Build history of the part. All positions in model axes, mm. A direction names the side the tool comes from. Round coordinates to 2 decimals unless told otherwise and drop trailing zeros. Write each loop counter-clockwise with the first axis right and the second up, starting at its lowest first coordinate (ties: lowest second). Pieces come first, ordered by that corner, then holes.
from build123d import *

# Parameters (mm, degrees)
SKETCH1_W                = 40
SKETCH1_H                = 20
BOSS_EXTRUDE1_DEPTH      = 29
SKETCH2_W                = 54
SKETCH2_H                = 20
BOSS_EXTRUDE2_DEPTH      = 2.5
SKETCH3_W                = 40
SKETCH3_H                = 20
BOSS_EXTRUDE3_DEPTH      = 5.5
BOSS_EXTRUDE4_DEPTH      = 2
SKETCH5_R                = 6
BOSS_EXTRUDE5_DEPTH      = 2
SKETCH6_R                = 3
BOSS_EXTRUDE6_DEPTH      = 4
SKETCH7_R                = 2.05
CUT_EXTRUDE2_DEPTH       = 4
BOSS_EXTRUDE8_DEPTH      = 0.5
BOSS_EXTRUDE8_DEPTH_BACK = 0.5


with BuildPart() as part:
    # Sketch1 → Boss-Extrude1 (new body)
    with BuildSketch(Plane(origin=(0, 0, 0), x_dir=(1, 0, 0), z_dir=(0, 1, 0))):
        Rectangle(SKETCH1_W, SKETCH1_H)
    extrude(amount=BOSS_EXTRUDE1_DEPTH)

    # Sketch2 → Boss-Extrude2 (add)
    with BuildSketch(Plane(origin=(0, 29, 0), x_dir=(1, 0, 0), z_dir=(0, 1, 0))):
        Rectangle(SKETCH2_W, SKETCH2_H)
    extrude(amount=BOSS_EXTRUDE2_DEPTH)

    # Sketch3 → Boss-Extrude3 (add)
    with BuildSketch(Plane(origin=(0, 31.5, 0), x_dir=(1, 0, 0), z_dir=(0, 1, 0))):
        Rectangle(SKETCH3_W, SKETCH3_H)
    extrude(amount=BOSS_EXTRUDE3_DEPTH)

    # Sketch4 → Boss-Extrude4 (add)
    with BuildSketch(Plane(origin=(0, 37, 0), x_dir=(1, 0, 0), z_dir=(0, 1, 0))):
        with BuildLine():
            Line((-10.302888497, 5.203858548), (-10.302888497, 8.863863335))
            Line((-10.302888497, 8.863863335), (6.370537096, 8.863863335))
            ThreePointArc((6.370537096, 8.863863335), (14.138323544, 9.494784112), (20, 4.358898944))
            Line((20, 4.358898944), (20, -4.358898944))
            ThreePointArc((20, -4.358898944), (14.138323544, -9.494784112), (6.370537096, -8.863863335))
            Line((6.370537096, -8.863863335), (-10.302888497, -8.863863335))
            Line((-10.302888497, -8.863863335), (-10.302888497, -5.203858548))
            ThreePointArc((-10.302888497, -5.203858548), (-12.798836729, 0), (-10.302888497, 5.203858548))
        make_face()
    extrude(amount=BOSS_EXTRUDE4_DEPTH)

    # Sketch5 → Boss-Extrude5 (add)
    with BuildSketch(Plane(origin=(0, 39, 0), x_dir=(1, 0, 0), z_dir=(0, 1, 0))):
        with Locations((11, 0)):
            Circle(SKETCH5_R)
    extrude(amount=BOSS_EXTRUDE5_DEPTH)

    # Sketch6 → Boss-Extrude6 (add)
    with BuildSketch(Plane(origin=(0, 41, 0), x_dir=(1, 0, 0), z_dir=(0, 1, 0))):
        with Locations((11, 0)):
            Circle(SKETCH6_R)
    extrude(amount=BOSS_EXTRUDE6_DEPTH)

    # Sketch7 → Cut-Extrude2 (cut)
    with BuildSketch(Plane(origin=(0, 31.5, 0), x_dir=(1, 0, 0), z_dir=(0, 1, 0))):
        with Locations((-25, 5)):
            Circle(SKETCH7_R)
        with Locations((-25, -5)):
            Circle(SKETCH7_R)
        with Locations((25, 5)):
            Circle(SKETCH7_R)
        with Locations((25, -5)):
            Circle(SKETCH7_R)
    extrude(amount=-CUT_EXTRUDE2_DEPTH, mode=Mode.SUBTRACT)

    # Sketch8 → Boss-Extrude8 (add, two sides)
    with BuildSketch(Plane.XY) as boss_extrude8_sk:
        Polygon((-20, 34), (-27, 31.5), (-20, 31.5), align=None)
        Polygon((20, 31.5), (20, 34), (27, 31.5), align=None)
    extrude(amount=BOSS_EXTRUDE8_DEPTH)
    extrude(boss_extrude8_sk.sketch, amount=-BOSS_EXTRUDE8_DEPTH_BACK)


solid = part.part
1) Slice it at B-B (x = 25). Write the cut outline in (y, z).
Results:
outline: (29, -10) - (31.5, -10) - (31.5, -7.05) - (29, -7.05) - close; (29, -2.95) - (31.5, -2.95) - (31.5, -0.5) - (32.21, -0.5) - (32.21, 0.5) - (31.5, 0.5) - (31.5, 2.95) - (29, 2.95) - close; (29, 7.05) - (31.5, 7.05) - (31.5, 10) - (29, 10) - close
2) Slice it at C-C (y = 11.5). Write the cut outline in (x, z).
Results:
outline: (-20, -10) - (20, -10) - (20, 10) - (-20, 10) - close
3) Slice it at D-D (x = 12.5). Write the cut outline in (y, z), plus the area to 3 significant figures.
Results:
outline: (0, -10) - (37, -10) - (37, -9.89) - (39, -9.89) - (39, -5.81) - (41, -5.81) - (41, -2.6) - (45, -2.6) - (45, 2.6) - (41, 2.6) - (41, 5.81) - (39, 5.81) - (39, 9.89) - (37, 9.89) - (37, 10) - (0, 10) - close
area: 824 mm2
4) Pin check, flat tips, straight feed: pin 1 Ø6.5 at (x, z) = (25, 5) entering from -Y; pin 2 Ø6.5 at (x, z) = (25, -5) entering from +Y; pin 3 Ø6 at (y, z) = (7.5, -0.5) entering from -X. Stop position of each tip, or through.
Results:
pin 1: stops at y = 29
pin 2: stops at y = 31.5
pin 3: stops at x = -20
5) Wall check: L1, parallel to Z at x = 25, y = 30.85; L2, parallel to X at y = 30.85, z = -5; L3, parallel to Y at x = -10.5, z = -6.5. Give the ranges that are in metal, low to high.
Results:
L1: z = -10 to -7.05, -2.95 to 2.95, 7.05 to 10
L2: x = -22.95 to 22.95
L3: y = 0 to 37
6) Which spindle directions (+Z, -Z, +X, -X, +Y, -Y) get a long thin tool onto all of the face, cutting with end or side? Do faces 1 (the cylindrical face through (14.03, 37.99, -9.53)), 2 (the flat face through (22.7, 31.5, -5.3)), 3 (the flat face through (-22.8, 31.5, -5.3)), 4 (the flat face through (8, 41, 1)). Say none if no direction does.
Results:
face 1: -Z, +Y
face 2: -Z, +X, +Y
face 3: -Z, -X, +Y
face 4: +Y
7) Slice it at A-A (x = -5). Write the cut outline in (y, z), plus the area to 3 significant figures.
Results:
outline: (0, -10) - (37, -10) - (37, -8.86) - (39, -8.86) - (39, 8.86) - (37, 8.86) - (37, 10) - (0, 10) - close
area: 775 mm2
8) Mould opens along X. For faces 5 (the flat face through (-10.303, 38, -7)), 6 (the cylindrical face through (-22.95, 30.27, 5.08)), 7 (the flat face through (-14, 37, 1)), 8 (the cylindrical face through (16.54, 39.99, 2.3)) say: released by +X, released by -X, zero draft, split by the parting line, or undercut.
Results:
face 5: released by -X
face 6: undercut
face 7: zero draft
face 8: split by the parting line
